Check sheet for the drawn part. Datum: minimum x, y, z corner. Units: mm. A direction names the side the tool comes from. Round coordinates to 2 decimals unless told otherwise and drop trailing zeros. Write each loop counter-clockwise with the first axis right and the second up, starting at its lowest first coordinate (ties: lowest second). Pieces come first, ordered by that corner, then holes. Notation, with made-up numbers: (63.25, 42) -> (79.25, 42) arc R16 cw to (79.25, 53) -> close; hole circle Ø8 at (73, 61). An arc over 180 degrees is marked (long way). Use a Markdown table: item, result.
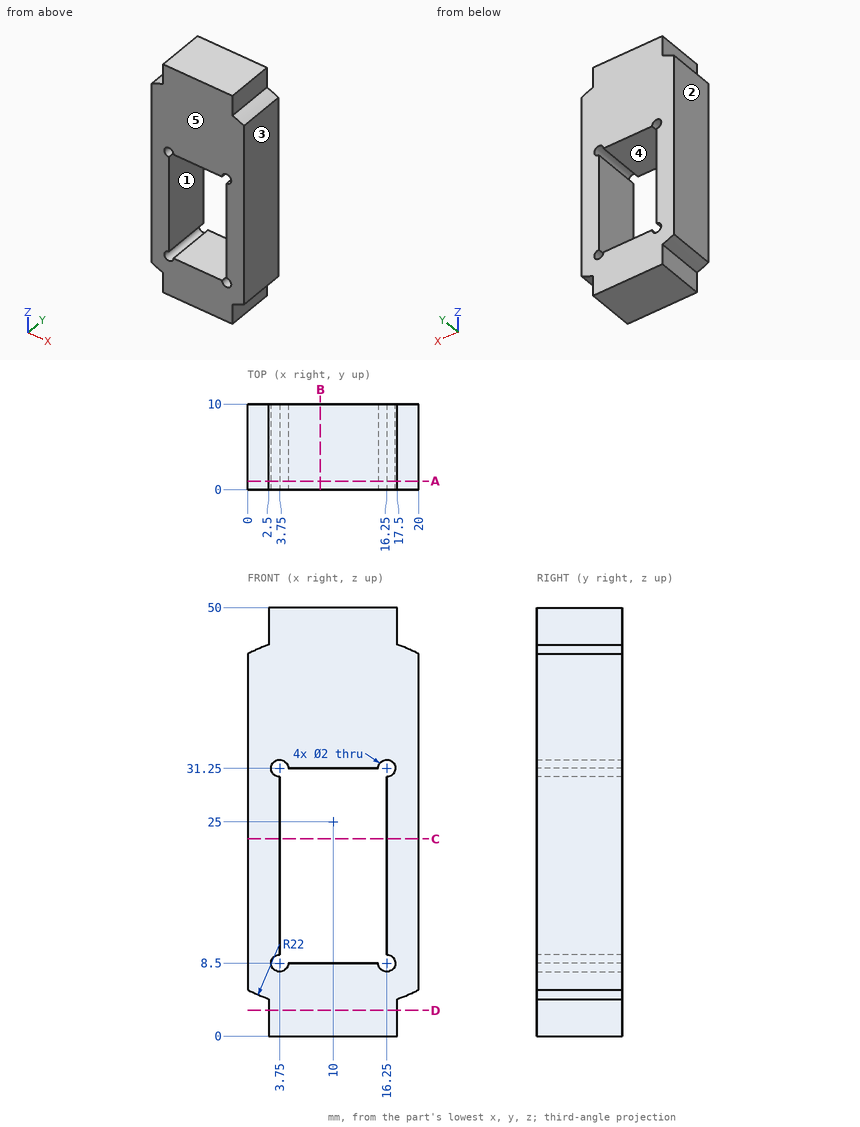
(1) Access from +Z, -Z, +X, -X, +Y, -Y to the whole of each face (thin tool, end or side, straight path). Record for the marked faces 1 and 2.
A:
| item | result |
|---|---|
| face 1 | +Y, -Y |
| face 2 | +Z, -Z, -X, +Y, -Y |
(2) Section check C-C on z = 23. Record the cut outline in (x, y), plus the area to 3 significant figures.
A:
| item | result |
|---|---|
| outline | (0, 0) -> (3.75, 0) -> (3.75, 10) -> (0, 10) -> close; (16.25, 0) -> (20, 0) -> (20, 10) -> (16.25, 10) -> close |
| area | 75.0 mm2 |
(3) Release check for a two-part mould opening along X. For the marked faces 3, 4 and 5 record: +X half, -X half, draft (parallel to the pull), parting line (faces both ways), or undercut.
A:
| item | result |
|---|---|
| face 3 | +X half |
| face 4 | undercut |
| face 5 | draft |
(4) Section check B-B on x = 8.5. Record the cut outline in (y, z), plus the area to 4 significant figures.
A:
| item | result |
|---|---|
| outline | (0, 0) -> (10, 0) -> (10, 8.5) -> (0, 8.5) -> close; (0, 31.25) -> (10, 31.25) -> (10, 50) -> (0, 50) -> close |
| area | 272.5 mm2 |
(5) Section check D-D on z = 3. Record the cut outline in (x, y), plus the area to 3 significant figures.
A:
| item | result |
|---|---|
| outline | (2.5, 0) -> (17.5, 0) -> (17.5, 10) -> (2.5, 10) -> close |
| area | 150 mm2 |
(6) Section check A-A on y = 1. Record the cut outline in (x, z), plus the area to 3 significant figures.
A:
| item | result |
|---|---|
| outline | (0, 5.4) arc R22 ccw to (2.5, 4.32) -> (2.5, 0) -> (17.5, 0) -> (17.5, 4.32) arc R22 ccw to (20, 5.4) -> (20, 44.6) arc R22 ccw to (17.5, 45.68) -> (17.5, 50) -> (2.5, 50) -> (2.5, 45.68) arc R22 ccw to (0, 44.6) -> close; hole (3.75, 9.5) arc R1 ccw (long way) to (4.75, 8.5) -> (15.25, 8.5) arc R1 ccw (long way) to (16.25, 9.5) -> (16.25, 30.25) arc R1 ccw (long way) to (15.25, 31.25) -> (4.75, 31.25) arc R1 ccw (long way) to (3.75, 30.25) -> close |
| area | 658 mm2 |
(7) Gauge pin test, flat ends, axial feed: pin 1 Ø2.5 at (x, z) = (3.75, 31.25) entering from -Y; pin 2 Ø4.5 at (y, z) = (6, 1.5) entering from -X; pin 3 Ø3.5 at (y, z) = (6.5, 47.5) entering from +X; pin 4 Ø1.8 at (x, z) = (16.25, 31.25) entering from -Y. Record the tip position at first contact, or that the pin passes through.
A:
| item | result |
|---|---|
| pin 1 | stops at y = 0 |
| pin 2 | stops at x = 2.5 |
| pin 3 | stops at x = 17.5 |
| pin 4 | passes through |
(8) Thickness scan on line 1 (Z direction, x = 13.75, y = 7); line 2 (X direction, y = 6, z = 31.5); line 3 (X direction, y = 6.75, z = 11.5). Record the ranges inside material, lowest first.
A:
| item | result |
|---|---|
| line 1 | z = 0 to 8.5, 31.25 to 50 |
| line 2 | x = 0 to 2.78, 4.72 to 15.28, 17.22 to 20 |
| line 3 | x = 0 to 3.75, 16.25 to 20 |
